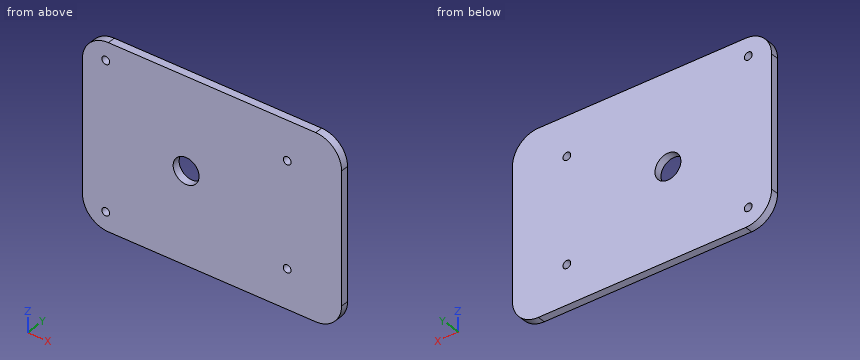
from build123d import *

# Parameters (mm, degrees)
SKETCH_1_W          = 100
SKETCH_1_H          = 70
EXTRUDE_1_DEPTH     = 3
FILLET_1_R          = 10
SKETCH_2_R          = 5
CUT_EXTRUDE_1_DEPTH = 70.526973183
SKETCH_3_R          = 1.5
CUT_EXTRUDE_2_DEPTH = 70.526973183


with BuildPart() as part:
    # 草图1 → 凸台-拉伸1 (new body)
    with BuildSketch(Plane(origin=(0, 0, 0), x_dir=(1, 0, 0), z_dir=(0, 1, 0))):
        with Locations((10, 0)):
            Rectangle(SKETCH_1_W, SKETCH_1_H)
    extrude(amount=EXTRUDE_1_DEPTH)

    # 圆角1
    fillet_1_edges = [part.edges().sort_by_distance(p)[0] for p in [
        (-40, 1.5, -35),
        (60, 1.5, -35),
        (60, 1.5, 35),
        (-40, 1.5, 35),
    ]]
    fillet(fillet_1_edges, radius=FILLET_1_R)

    # 草图2 → 切除-拉伸1 (cut, through all)
    with BuildSketch(Plane(origin=(0, 3, 0), x_dir=(1, 0, 0), z_dir=(0, 1, 0))):
        with Locations(Location((0, 0, 0), (0, 0, 270))):
            Circle(SKETCH_2_R)
    extrude(amount=-CUT_EXTRUDE_1_DEPTH, mode=Mode.SUBTRACT)

    # 草图3 → 切除-拉伸2 (cut, through all)
    with BuildSketch(Plane(origin=(0, 3, 0), x_dir=(1, 0, 0), z_dir=(0, 1, 0))):
        with Locations(Location((-31, 28, 0), (0, 0, 270))):
            Circle(SKETCH_3_R)
        with Locations(Location((39, 20, 0), (0, 0, 270))):
            Circle(SKETCH_3_R)
    cut_extrude_2 = extrude(amount=-CUT_EXTRUDE_2_DEPTH, mode=Mode.SUBTRACT)

    # 镜向1: 切除-拉伸2 across plane
    add(cut_extrude_2.mirror(Plane.XY), mode=Mode.SUBTRACT)


solid = part.part
Check sheet for the modelled part. Datum: model origin and axes. Units: mm. Give positions to 0.01 mm unless a question says otherwise; leave off trailing zeros. Loops run counter-clockwise (first coordinate to the right, second up) from the corner with the lowest first, then second, coordinate; pieces in that order, holes last. Notation, with made-up numbers: M 74.25,34 L 99.25,34 A32 cw 99.25,73 Z; hole C 87,52 d8. An arc over 180 degrees is marked long. Answer as a JSON object with one key per item and string values. Group by question number.
Q1. Go/stop test with a flat-tipped pin: P1, Ø1.8, axis at x = -31, z = -28, coming from the -Y side. Record where the tip stops, or that it passes through.
Q2. Cross-section at C-C on y = 1.05. Record the cut outline in (x, z), then the cut area to 3 significant figures.
Q3. Cross-section at A-A on x = 39. Record the cut outline in (y, z), then the cut area to 3 significant figures.
Q4. Material ranges on line 1 along X through (y, z) = (2.35, 0); line 2 along X through (y, z) = (0.65, -20); line 3 along Z through (x, y) = (1.5, 2.6), recorded low to high. Write a range as [from, to].
Q5. Cross-section at D-D on x = 0. Record the cut outline in (y, z).
Q6. Cross-section at B-B on z = 0. Record the cut outline in (x, y).
Evaluation:
{
 "1": {"P1": "passes through"},
 "2": {"outline": "M -40,-25 A10 ccw -30,-35 L 50,-35 A10 ccw 60,-25 L 60,25 A10 ccw 50,35 L -30,35 A10 ccw -40,25 Z; hole C -31,-28 d3; hole C -31,28 d3; hole C 0,0 d10; hole C 39,-20 d3; hole C 39,20 d3", "area": "6,810 mm2"},
 "3": {"outline": "M 0,-35 L 3,-35 L 3,-21.5 L 0,-21.5 Z; M 0,-18.5 L 3,-18.5 L 3,18.5 L 0,18.5 Z; M 0,21.5 L 3,21.5 L 3,35 L 0,35 Z", "area": "192 mm2"},
 "4": {"line 1": "x = [-40, -5], [5, 60]", "line 2": "x = [-40, 37.5], [40.5, 60]", "line 3": "z = [-35, -4.77], [4.77, 35]"},
 "5": {"outline": "M 0,-35 L 3,-35 L 3,-5 L 0,-5 Z; M 0,5 L 3,5 L 3,35 L 0,35 Z"},
 "6": {"outline": "M -40,0 L -5,0 L -5,3 L -40,3 Z; M 5,0 L 60,0 L 60,3 L 5,3 Z"}
}
